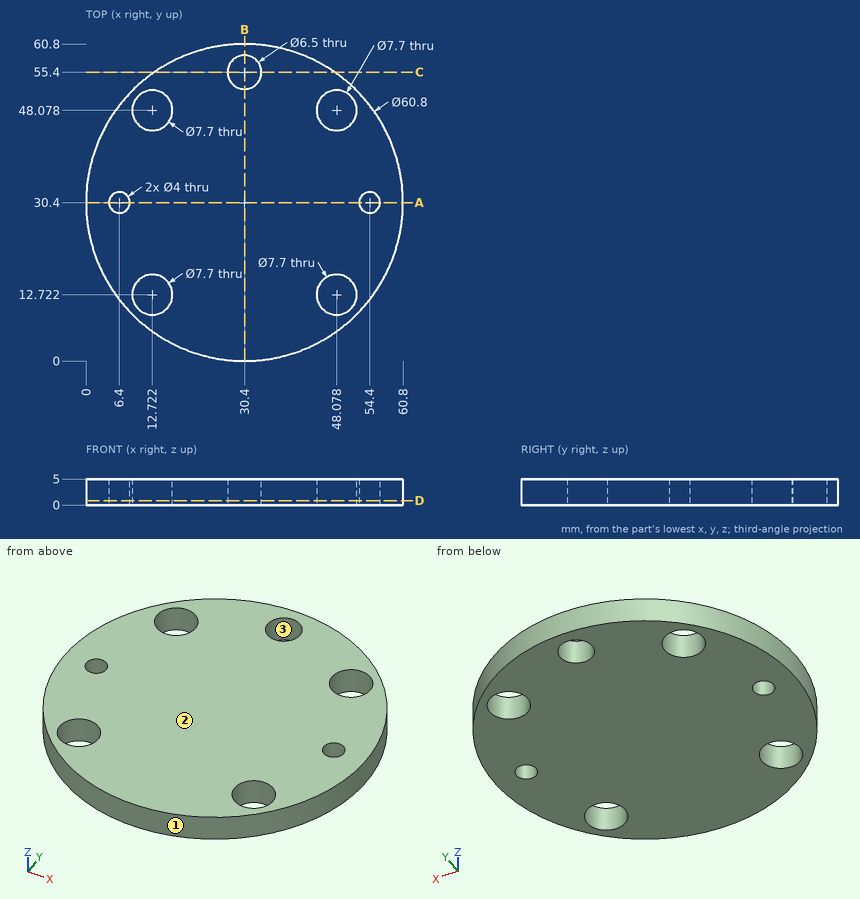
Study the drawing (mm; zero at the part's minimum x, y, z) and answer. Give positions to 0.01 mm unless a question says otherwise; leave off trailing zeros. Write each loop counter-clockwise with the first axis right and the second up, starting at its lowest first coordinate (ties: lowest second). Pieces come first, ordered by that corner, then holes. Notation, with made-up numbers: (7, -29.75) - (45, -29.75) arc R22 cw to (45, -0.75) - close; hole circle Ø10 at (35.5, 16). An arc over 180 degrees is marked (long way). Write item = value, one per line. Start each with the question number.
Item 1: The mould has two halves that part along Y. Classify the marked faces 1, 2 and 3: +Y half, -Y half, draft (parallel to the pull), parting line (faces both ways), or undercut.
Item 2: Find the intervals of material crossed by probe 1 along X at (y, z) = (13.5, 4.5); probe 2 along Y at (x, z) = (10, 1.95) (1 decimal), in increasing order. Write a range as [from, to].
Item 3: Find section A-A (y = 30.4). Give the vertices of the cut face in (x, z).
Item 4: Each of these flat-tipped pins is pushed along its axis until it touches: P1, Ø2, axis at y = 11, z = 2.5, coming from the +X side; P2, Ø1.5, axis at y = 42, z = 3.5, coming from the +X side. Where does it stop, or does it pass through?
Item 5: Find section B-B (x = 30.4). Give the vertices of the cut face in (y, z).
Item 6: Find section D-D (z = 0.85). Give the vertices of the cut face in (x, y), then the cut area to 3 significant figures.
Item 7: Find section C-C (y = 55.4). Give the vertices of the cut face in (x, z).
Response:
q1.face_1 = parting line
q1.face_2 = draft
q1.face_3 = undercut
q2.probe_1 = [5.13, 8.95], [16.49, 44.31], [51.85, 55.67]
q2.probe_2 = [7.9, 10], [15.4, 45.4], [50.8, 52.9]
q3.outline = (0, 0) - (4.4, 0) - (4.4, 5) - (0, 5) - close; (8.4, 0) - (52.4, 0) - (52.4, 5) - (8.4, 5) - close; (56.4, 0) - (60.8, 0) - (60.8, 5) - (56.4, 5) - close
q4.P1 = 54.6
q4.P2 = 58.8
q5.outline = (0, 0) - (52.15, 0) - (52.15, 5) - (0, 5) - close; (58.65, 0) - (60.8, 0) - (60.8, 5) - (58.65, 5) - close
q6.outline = circle Ø60.8 at (30.4, 30.4); hole circle Ø4 at (6.4, 30.4); hole circle Ø7.7 at (12.72, 12.72); hole circle Ø7.7 at (12.72, 48.08); hole circle Ø6.5 at (30.4, 55.4); hole circle Ø7.7 at (48.08, 12.72); hole circle Ø7.7 at (48.08, 48.08); hole circle Ø4 at (54.4, 30.4)
q6.area = 2,660 mm²
q7.outline = (13.1, 0) - (27.15, 0) - (27.15, 5) - (13.1, 5) - close; (33.65, 0) - (47.7, 0) - (47.7, 5) - (33.65, 5) - close
